Design review of the part shown in the three views and the two pictorial views. Dimensions are in mm from the part's minimum x, y and z. A direction names the side the tool comes from. Give positions to 0.01 mm unless a question says otherwise; leave off trailing zeros. Loops run counter-clockwise (first coordinate to the right, second up) from the corner with the lowest first, then second, coordinate; pieces in that order, holes last.
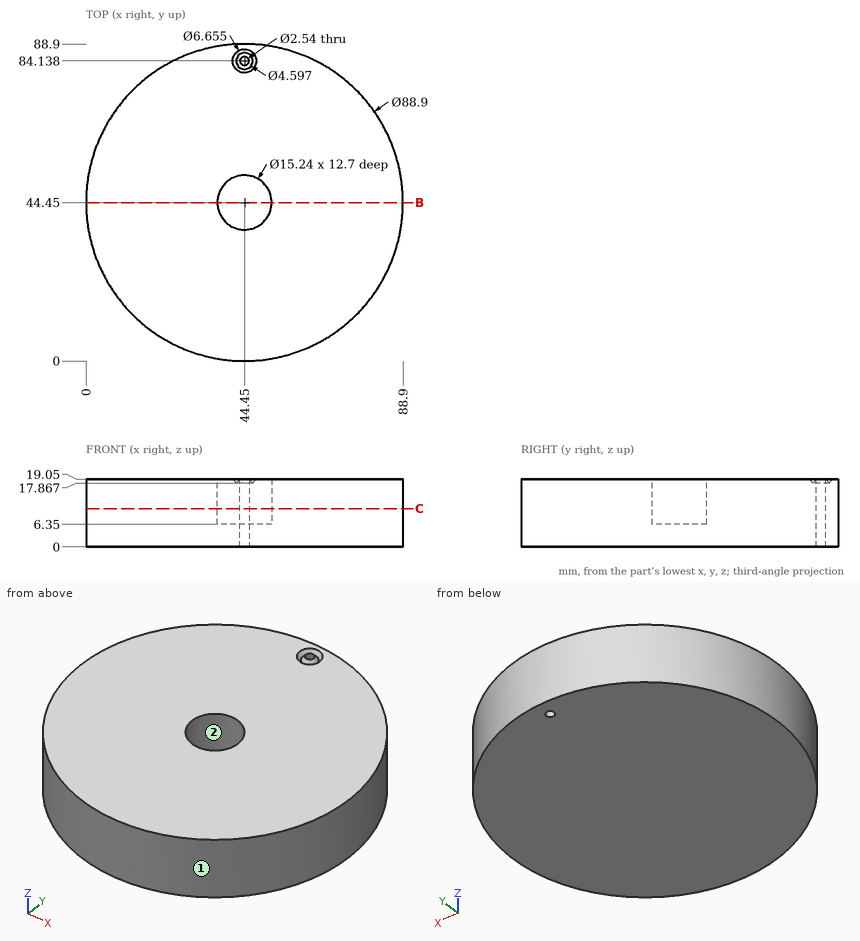
Q1. Consider section B-B on y = 44.45. Give the boundary of the cut face in (x, z), plus the area to 3 significant figures.
Answers:
outline: (0, 0) - (88.9, 0) - (88.9, 19.05) - (52.07, 19.05) - (52.07, 6.35) - (36.83, 6.35) - (36.83, 19.05) - (0, 19.05) - close
area: 1,500 mm2
Q2. For probe 1 along Y at (x, z) = (44.45, 14); probe 2 along X at (y, z) = (50.5, 6.5) (1 decimal); probe 3 along Y at (x, z) = (44.45, 5), list the stretches that pass through material, from the lowest coordinate up.
Answers:
probe 1: y = 0 to 36.83, 52.07 to 82.87, 85.41 to 88.9
probe 2: x = 0.4 to 39.8, 49.1 to 88.5
probe 3: y = 0 to 82.87, 85.41 to 88.9
Q3. For pin 1 Ø8 at (x, z) = (41.5, 6.5) entering from +Y; pin 2 Ø10 at (x, z) = (14, 11.5) entering from -Y; pin 3 Ø1 at (y, z) = (46, 7) entering from +X, all flat-tipped, find the tip position at first contact; note any pin that passes through.
Answers:
pin 1: stops at y = 88.9
pin 2: stops at y = 8.01
pin 3: stops at x = 88.89
Q4. Consider section C-C on z = 10.75. Give the boundary of the cut face in (x, y), plus the area to 3 significant figures.
Answers:
outline: circle Ø88.9 at (44.45, 44.45); hole circle Ø15.24 at (44.45, 44.45); hole circle Ø2.54 at (44.45, 84.14)
area: 6,020 mm2
Q5. Machinability: for the marked faces 1 and 2, which of the approach directions +Z, -Z, +X, -X, +Y, -Y give a long, thin tool a straight path to every point of the face, cutting with its end or side? Answer none if there is none.
Answers:
face 1: +Z, -Z
face 2: +Z
